```python
from build123d import *

# Parameters (mm, degrees)
SKETCH1_R           = 1.5
BOSS_EXTRUDE1_DEPTH = 3
FILLET2_R           = 1


with BuildPart() as part:
    # Sketch1 → Boss-Extrude1 (new body)
    with BuildSketch(Plane.XY):
        with BuildLine():
            Line((-2.5, 0), (-2.5, 25.6))
            ThreePointArc((-2.5, 25.6), (0, 28.1), (2.5, 25.6))
            Line((2.5, 25.6), (2.5, 0))
            ThreePointArc((2.5, 0), (0, -2.5), (-2.5, 0))
        make_face()
        with Locations((0, 25.6)):
            Circle(SKETCH1_R, mode=Mode.SUBTRACT)
        Circle(SKETCH1_R, mode=Mode.SUBTRACT)
    extrude(amount=BOSS_EXTRUDE1_DEPTH)

    # Fillet2
    # the kernel refuses this fillet: 1 mm, written as the material it takes off along each edge
    with BuildSketch(Plane(origin=(0, 0, 3), x_dir=(1, 0, 0), z_dir=(0, 1, 0))) as fillet2_piece_1:
        with BuildLine():
            CenterArc((2.5 - FILLET2_R, FILLET2_R), FILLET2_R, 270, 90)
            Line((2.5 - FILLET2_R, 0), (2.5, 0))
            Line((2.5, 0), (2.5, FILLET2_R))
        make_face()
    revolve(axis=Axis((0, 0, 3), (0, 0, -1)), revolution_arc=180, mode=Mode.SUBTRACT)
    with BuildSketch(Plane(origin=(0, 0, 0), x_dir=(1, 0, 0), z_dir=(0, 1, 0))) as fillet2_piece_2:
        with BuildLine():
            CenterArc((2.5 - FILLET2_R, -FILLET2_R), FILLET2_R, 0, 90)
            Line((2.5 - FILLET2_R, 0), (2.5, 0))
            Line((2.5, 0), (2.5, -FILLET2_R))
        make_face()
    revolve(axis=Axis((0, 0, 0), (0, 0, -1)), revolution_arc=180, mode=Mode.SUBTRACT)
    with BuildSketch(Plane(origin=(2.5, 25.6, 3), x_dir=(0, 0, -1), z_dir=(0, -1, 0)), Plane(origin=(-2.5, 0, 3), x_dir=(0, 0, -1), z_dir=(0, 1, 0))) as fillet2_piece_3:
        with BuildLine():
            CenterArc((FILLET2_R, -FILLET2_R), FILLET2_R, 90, 90)
            Line((0, -FILLET2_R), (0, 0))
            Line((0, 0), (FILLET2_R, 0))
        make_face()
    extrude(amount=25.6, mode=Mode.SUBTRACT)
    with BuildSketch(Plane(origin=(2.5, 25.6, 0), x_dir=(0, 0, 1), z_dir=(0, -1, 0)), Plane(origin=(-2.5, 0, 0), x_dir=(0, 0, 1), z_dir=(0, 1, 0))) as fillet2_piece_4:
        with BuildLine():
            CenterArc((FILLET2_R, FILLET2_R), FILLET2_R, 180, 90)
            Line((0, FILLET2_R), (0, 0))
            Line((0, 0), (FILLET2_R, 0))
        make_face()
    extrude(amount=25.6, mode=Mode.SUBTRACT)
    with BuildSketch(Plane(origin=(0, 25.6, 3), x_dir=(-1, 0, 0), z_dir=(0, -1, 0))) as fillet2_piece_5:
        with BuildLine():
            CenterArc((2.5 - FILLET2_R, FILLET2_R), FILLET2_R, 270, 90)
            Line((2.5 - FILLET2_R, 0), (2.5, 0))
            Line((2.5, 0), (2.5, FILLET2_R))
        make_face()
    revolve(axis=Axis((0, 25.6, 3), (0, 0, -1)), revolution_arc=180, mode=Mode.SUBTRACT)
    with BuildSketch(Plane(origin=(0, 25.6, 0), x_dir=(-1, 0, 0), z_dir=(0, -1, 0))) as fillet2_piece_6:
        with BuildLine():
            CenterArc((2.5 - FILLET2_R, -FILLET2_R), FILLET2_R, 0, 90)
            Line((2.5 - FILLET2_R, 0), (2.5, 0))
            Line((2.5, 0), (2.5, -FILLET2_R))
        make_face()
    revolve(axis=Axis((0, 25.6, 0), (0, 0, -1)), revolution_arc=180, mode=Mode.SUBTRACT)
    with BuildSketch(Plane(origin=(0, 25.6, 0), x_dir=(1, 0, 0), z_dir=(0, -1, 0))) as fillet2_piece_7:
        with BuildLine():
            CenterArc((1.5 + FILLET2_R, FILLET2_R), FILLET2_R, 180, 90)
            Line((1.5 + FILLET2_R, 0), (1.5, 0))
            Line((1.5, 0), (1.5, FILLET2_R))
        make_face()
    revolve(axis=Axis((0, 25.6, 0), (0, 0, 1)), mode=Mode.SUBTRACT)
    with BuildSketch(Plane(origin=(0, 25.6, 3), x_dir=(1, 0, 0), z_dir=(0, -1, 0))) as fillet2_piece_8:
        with BuildLine():
            CenterArc((1.5 + FILLET2_R, -FILLET2_R), FILLET2_R, 90, 90)
            Line((1.5 + FILLET2_R, 0), (1.5, 0))
            Line((1.5, 0), (1.5, -FILLET2_R))
        make_face()
    revolve(axis=Axis((0, 25.6, 3), (0, 0, 1)), mode=Mode.SUBTRACT)
    with BuildSketch(Plane(origin=(0, 0, 0), x_dir=(1, 0, 0), z_dir=(0, -1, 0))) as fillet2_piece_9:
        with BuildLine():
            CenterArc((1.5 + FILLET2_R, FILLET2_R), FILLET2_R, 180, 90)
            Line((1.5 + FILLET2_R, 0), (1.5, 0))
            Line((1.5, 0), (1.5, FILLET2_R))
        make_face()
    revolve(axis=Axis((0, 0, 0), (0, 0, 1)), mode=Mode.SUBTRACT)
    with BuildSketch(Plane(origin=(0, 0, 3), x_dir=(1, 0, 0), z_dir=(0, -1, 0))) as fillet2_piece_10:
        with BuildLine():
            CenterArc((1.5 + FILLET2_R, -FILLET2_R), FILLET2_R, 90, 90)
            Line((1.5 + FILLET2_R, 0), (1.5, 0))
            Line((1.5, 0), (1.5, -FILLET2_R))
        make_face()
    revolve(axis=Axis((0, 0, 3), (0, 0, 1)), mode=Mode.SUBTRACT)


solid = part.part
```
Could you check a few things on this model? Use its own coordinates, in mm. Round coordinates to 2 decimals unless told otherwise and drop trailing zeros. Write each loop counter-clockwise with the first axis right and the second up, starting at its lowest first coordinate (ties: lowest second). Pieces come first, ordered by that corner, then holes. Notation, with made-up numbers: M -13.5,13.5 L 42.5,13.5 A27 cw 42.5,51.5 Z; hole C 9,19 d6. An arc over 180 degrees is marked long. Write each question's results on one line, items separated by ' | '. Start each with the question number.
1. Imagine slicing it at B-B on y = 21.5. List the corners of the cut face in (x, z) for me.
2. Thinking about a two-plate mould opening in Y: for faces 1 (the face through (-0.1, 28.1, 1.5)), 2 (the face through (2.215, 12.979, 2.699)), 3 (the face through (-1.5, 0.07, 1.49)), 4 (the face through (-1.11, 26.61, 1.49)), which applies, +Y half, -Y half, draft (parallel to the pull), parting line (faces both ways), or undercut?
3. Imagine slicing it at A-A on x = 0. List the corners of the cut face in (y, z) for me, and give its area (3 significant figures).
4. Imagine slicing it at D-D on z = 2.25. List the corners of the cut face in (x, y) for me, and give its area (3 significant figures).
5. I'm going to push flat-ended pins straight in: pin 1 Ø2.5 at (x, y) = (0, 25.6) entering from +Z; pin 2 Ø3 at (x, y) = (-1.5, 24) entering from +Z. Where does each tip first touch, or does it pass through?
6. Imagine slicing it at C-C on z = 0.6. List the corners of the cut face in (x, y) for me.
7. I need wall thicknesses on L1, parallel to Y at x = 0, z = 1.55; L2, parallel to X at y = 0, z = 0.5; L3, parallel to Y at x = 0.9, z = 1.9. Which ranges of each line are inside material? Lowest first, please. Write a range as from..to.
Result sheet:
1) outline: M -2.5,1 A1 ccw -1.5,0 L 1.5,0 A1 ccw 2.5,1 L 2.5,2 A1 ccw 1.5,3 L -1.5,3 A1 ccw -2.5,2 Z
2) face 1: +Y half | face 2: draft | face 3: undercut | face 4: undercut
3) outline: M -2.5,1 A1 ccw -2,0.13 A1 ccw -1.5,1 L -1.5,2 A1 ccw -2,2.87 A1 ccw -2.5,2 Z; M 1.5,1 A1 ccw 2.5,0 L 23.1,0 A1 ccw 24.1,1 L 24.1,2 A1 ccw 23.1,3 L 2.5,3 A1 ccw 1.5,2 Z; M 27.1,1 A1 ccw 27.6,0.13 A1 ccw 28.1,1 L 28.1,2 A1 ccw 27.6,2.87 A1 ccw 27.1,2 Z | area: 71.4 mm^2
4) outline: M -2.47,0 A2.47 ccw 2.47,0 L 2.47,25.6 A2.47 ccw -2.47,25.6 Z; hole C 0,0 d3.06; hole C 0,25.6 d3.06 | area: 131 mm^2
5) pin 1: passes through | pin 2: stops at z = 3
6) outline: M -2.42,0 A2.42 ccw 2.42,0 L 2.42,25.6 A2.42 ccw -2.42,25.6 Z; hole C 0,0 d3.17; hole C 0,25.6 d3.17
7) L1: y = -2.5..-1.5, 1.5..24.1, 27.1..28.1 | L2: x = -2.37..-1.63, 1.63..2.37 | L3: y = -2.33..-1.2, 1.2..24.4, 26.8..27.93
